```python
from build123d import *

# Parameters (mm, degrees)
SKETCH1_W = 15
SKETCH1_H = 2.5
FILLET1_R = 0.4
SKETCH2_W = 1.1
SKETCH2_H = 0.2


with BuildPart() as part:
    # Sketch1 → Revolve1 (revolve)
    with BuildSketch(Plane.XY):
        with Locations((7.5, 3.75)):
            Rectangle(SKETCH1_W, SKETCH1_H)
    revolve(axis=Axis((0, 0, 0), (1, 0, 0)))

    # Fillet1
    fillet1_edges = [part.edges().sort_by_distance(p)[0] for p in [
        (0, -5, 0),
        (15, -5, 0),
    ]]
    fillet(fillet1_edges, radius=FILLET1_R)

    # Sketch2 → Cut-Revolve1 (revolve, cut)
    with BuildSketch(Plane.XY):
        with Locations((12.05, 4.9)):
            Rectangle(SKETCH2_W, SKETCH2_H)
        with Locations((2.95, 4.9)):
            Rectangle(SKETCH2_W, SKETCH2_H)
    revolve(axis=Axis((15, 0, 0), (-1, 0, 0)), mode=Mode.SUBTRACT)


solid = part.part
```
Work out the finished part from the listing and answer in its coordinate system (mm). A direction names the side the tool comes from. Round coordinates to 2 decimals unless told otherwise and drop trailing zeros. Loops run counter-clockwise (first coordinate to the right, second up) from the corner with the lowest first, then second, coordinate; pieces in that order, holes last. Notation, with made-up numbers: M -19.75,74.25 L 22.25,74.25 A11 ccw 22.25,83.25 Z; hole C 54,54.25 d7. An arc over 180 degrees is marked long. Use CSV: the item, a comma, the result in double quotes.
Q1. The mould has two halves that part along X. Classify faces 3 (the cylindrical face through (7.56, -1.08, -4.88)), 4 (the flat face through (0, -2, -2)), 5 (the flat face through (15, -2, -2)), 6 (the cylindrical face through (12.06, 2.58, -4.05)): pulls with the +X half, pulls with the -X half, needs draft (parallel to the pull), parting line crosses it, or undercut.
Determined:
face 3,"needs draft"
face 4,"pulls with the -X half"
face 5,"pulls with the +X half"
face 6,"undercut"
Q2. Section D-D, the plane x = 2.75 is taken. Determine the outline of the cut face in (y, z).
Determined:
outline,"C 0,0 d9.6; hole C 0,0 d5"
Q3. Consider L1, parallel to Z at x = 6, y = 0; L2, parallel to Z at x = 11.75, y = 0; L3, parallel to Y at x = 2.5, z = 0.25. Determine where each line is inside the solid, lowest interval first.
Determined:
L1,"-5 to -2.5, 2.5 to 5"
L2,"-4.8 to -2.5, 2.5 to 4.8"
L3,"-4.79 to -2.49, 2.49 to 4.79"
Q4. Section A-A, the plane z = 0 is taken. Determine the outline of the cut face in (x, y), then the cut area to 3 significant figures.
Determined:
outline,"M 0,-4.6 A0.4 ccw 0.4,-5 L 2.4,-5 L 2.4,-4.8 L 3.5,-4.8 L 3.5,-5 L 11.5,-5 L 11.5,-4.8 L 12.6,-4.8 L 12.6,-5 L 14.6,-5 A0.4 ccw 15,-4.6 L 15,-2.5 L 0,-2.5 Z; M 0,2.5 L 15,2.5 L 15,4.6 A0.4 ccw 14.6,5 L 12.6,5 L 12.6,4.8 L 11.5,4.8 L 11.5,5 L 3.5,5 L 3.5,4.8 L 2.4,4.8 L 2.4,5 L 0.4,5 A0.4 ccw 0,4.6 Z"
area,"74.0 mm2"
Q5. Section C-C, the plane x = 13 is taken. Determine the outline of the cut face in (y, z), then the cut area to 3 significant figures.
Determined:
outline,"C 0,0 d10; hole C 0,0 d5"
area,"58.9 mm2"
Q6. A tool of negligible diameter and unlimited length cuts with its end or side. For faces 1 (the cylindrical face through (2.96, 2.58, -4.05)), 2 (the cylindrical face through (7.6, -0.54, -2.44)), from which of +Z, -Z, +X, -X, +Y, -Y can it reach the whole face along a straight path? Write none if from no direction.
Determined:
face 1,"none"
face 2,"+X, -X"
Q7. Each of these flat-tipped pins is pushed along its axis until it touches: pin 1 (1 mm diameter, centred on y = 0.5, z = -1, fed in from -X); pin 2 (4 mm diameter, centred on x = 12, y = 2.5, fed in from -Z); pin 3 (4 mm diameter, centred on x = 6, z = 2.5, fed in from -Y). Where does it stop, or does it pass through?
Determined:
pin 1,"through"
pin 2,"z = -4.97"
pin 3,"y = -4.97"
